```python
from build123d import *

# Parameters (mm, degrees)
SKETCH1_R               = 3
BOSS_EXTRUDE1_DEPTH     = 11.5
SKETCH4_R               = 1
BOSS_EXTRUDE2_DEPTH     = 5
SKETCH9_R               = 1
CUT_EXTRUDE1_DEPTH      = 4
CUT_EXTRUDE1_DEPTH_BACK = 4
CHAMFER1_SIZE           = 0.25
CHAMFER2_SIZE           = 0.25
CHAMFER3_SIZE           = 0.125


with BuildPart() as part:
    # Sketch1 → Boss-Extrude1 (new body)
    with BuildSketch(Plane(origin=(0, 0, 0), x_dir=(1, 0, 0), z_dir=(0, 1, 0))):
        Circle(SKETCH1_R)
    extrude(amount=BOSS_EXTRUDE1_DEPTH)

    # Sketch4 → Boss-Extrude2 (add)
    with BuildSketch(Plane(origin=(0, 11.5, 0), x_dir=(1, 0, 0), z_dir=(0, 1, 0))):
        with Locations((0, -1.5)):
            Circle(SKETCH4_R)
    extrude(amount=BOSS_EXTRUDE2_DEPTH)

    # Sketch9 → Cut-Extrude1 (cut, two sides)
    with BuildSketch(Plane(origin=(0, 0, 0), x_dir=(0, 0, -1), z_dir=(1, 0, 0))) as cut_extrude1_sk:
        with Locations((0, 2.5)):
            Circle(SKETCH9_R)
    extrude(amount=CUT_EXTRUDE1_DEPTH, mode=Mode.SUBTRACT)
    extrude(cut_extrude1_sk.sketch, amount=-CUT_EXTRUDE1_DEPTH_BACK, mode=Mode.SUBTRACT)

    # Chamfer1
    chamfer1_edges = [part.edges().sort_by_distance(p)[0] for p in [
        (-3, 11.5, 0),
    ]]
    chamfer(chamfer1_edges, length=CHAMFER1_SIZE)

    # Chamfer2
    chamfer2_edges = [part.edges().sort_by_distance(p)[0] for p in [
        (-3, 0, 0),
    ]]
    chamfer(chamfer2_edges, length=CHAMFER2_SIZE)

    # Chamfer3
    chamfer3_edges = [part.edges().sort_by_distance(p)[0] for p in [
        (-1, 16.5, 1.5),
    ]]
    chamfer(chamfer3_edges, length=CHAMFER3_SIZE)


solid = part.part
```
Input: part model. Units: mm. Frame: model coordinates. A direction names the side the tool comes from. Give positions to 0.01 mm unless a question says otherwise; leave off trailing zeros. Write each loop counter-clockwise with the first axis right and the second up, starting at its lowest first coordinate (ties: lowest second). Pieces come first, ordered by that corner, then holes. Notation, with made-up numbers: (-25, 78.25) - (12, 78.25) arc R10 cw to (12, 96.25) - close; hole circle Ø9 at (-32.5, 46.5). An arc over 180 degrees is marked (long way). Write item = value, one per line. Start each with the question number.
1. Ray query, L1, parallel to Y at x = -0.25, z = 0; L2, parallel to X at y = 15.75, z = 1.5; L3, parallel to Y at x = 1.25, z = -2. Return the intervals inside material, ascending.
2. Section query A-A, the plane z = 0. Output: boundary loops of the cut face in (x, y), then the cut area to 3 significant figures.
3. Section query C-C, the plane y = 3.25. Output: boundary loops of the cut face in (x, z).
4. First-contact query: pin 1 Ø1.8 at (y, z) = (2.5, 0) entering from -X; pin 2 Ø2 at (x, y) = (-0.5, 7.5) entering from +Z. Flat tips, straight axial feed; report the tip coordinate or a pass-through.
5. Access query for faces 1 (the cylindrical face through (-0.217, 13.903, 2.476)), 2 (the cylindrical face through (2.77, 5.67, 1.15)). Directions: +Z, -Z, +X, -X, +Y, -Y. A direction counts if a zero-diameter tool reaches every point of the face in a straight line with its end or side. Return the directions, or none.
6. Section query D-D, the plane y = 12. Output: boundary loops of the cut face in (x, z), then the cut area to 3 significant figures.
7. Section query B-B, the plane y = 9. Output: boundary loops of the cut face in (x, z), then the cut area to 3 significant figures.
Check sheet entries:
q1.L1 = 0 to 1.5, 3.5 to 11.5
q1.L2 = -1 to 1
q1.L3 = 0 to 11.5
q2.outline = (-3, 0.25) - (-2.75, 0) - (2.75, 0) - (3, 0.25) - (3, 1.5) - (-3, 1.5) - close; (-3, 3.5) - (3, 3.5) - (3, 11.25) - (2.75, 11.5) - (-2.75, 11.5) - (-3, 11.25) - close
q2.area = 56.9 mm2
q3.outline = (-2.93, -0.66) arc R3 ccw to (2.93, -0.66) - close; (-2.93, 0.66) - (2.93, 0.66) arc R3 ccw to start
q4.pin_1 = through
q4.pin_2 = 3
q5.face_1 = +Y
q5.face_2 = +Y, -Y
q6.outline = circle Ø2 at (0, 1.5)
q6.area = 3.14 mm2
q7.outline = circle Ø6 at (0, 0)
q7.area = 28.3 mm2
